```python
from build123d import *

# Parameters (mm, degrees)
F0_W           = 64
F0_H           = 25
F1_DEPTH       = 3
F3_D           = 3.3
F3_CSINK_D     = 6.72
F3_CSINK_ANGLE = 90
F4_R           = 5


with BuildPart() as f1:
    # F0 (on Front) → F1 (new body)
    with BuildSketch(Plane.XZ):
        with Locations((32, 12.5)):
            Rectangle(F0_W, F0_H)
    extrude(amount=F1_DEPTH)

    # F3 (through all)
    with Locations(Plane.XZ.offset(3)):
        with Locations((3, 21.5), (28, 21.5), (28, 3.5), (3, 3.5)):
            CounterSinkHole(F3_D / 2, F3_CSINK_D / 2, counter_sink_angle=F3_CSINK_ANGLE)

    # F4
    f4_edges = [f1.edges().sort_by_distance(p)[0] for p in [
        (64, -1.5, 0),
        (64, -1.5, 25),
    ]]
    fillet(f4_edges, radius=F4_R)


solid = f1.part
```
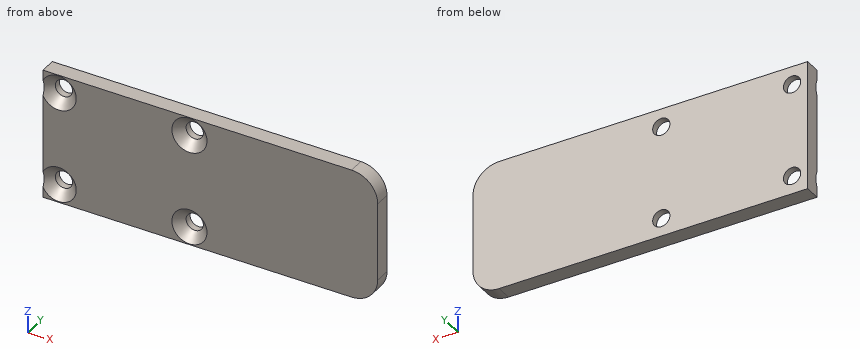
Could you check a few things on this model? Use its own coordinates, in mm. Coordinates: 2 decimals unless noted, no trailing zeros. Order: outer loops, then holes, each group sorted by start corner. A loop starts at its lowest first (then second) coordinate and runs counter-clockwise, first axis right, second up. Notation, with made-up numbers: M 50,34.25 L 82,34.25 A34 cw 82,71.25 Z; hole C 12,72.5 d1. An arc over 180 degrees is marked long. Use one line per item in the form item = value. Start each with the question number.
1. Suppose I cut it at B-B on z = 21.5. Write out the boundary of the cut face in (x, y).
2. Suppose I cut it at A-A on x = 3. Write out the boundary of the cut face in (y, z), then the cut area to 3 significant figures.
3. Please list where these lines run through material, in increasing order: line 1 (Z direction, x = 3, y = -0.95); line 2 (X direction, y = -2.2, z = 22.75); line 3 (X direction, y = -0.75, z = 3.5).
4. For pin 1 (3 mm diameter, centred on x = 28, z = 21.5, fed in from +Y); pin 2 (4 mm diameter, centred on x = 3, z = 3.5, fed in from -Y); pin 3 (5.5 mm diameter, centred on x = 3, z = 21.5, fed in from -Y), each with a flat end and sliding along its axis, tell me the tip position at first contact or that it passes through.
Geometry says:
q1.outline = M 0,-2.64 L 1.35,-1.29 L 1.35,0 L 0,0 Z; M 4.65,-1.29 L 6.36,-3 L 24.64,-3 L 26.35,-1.29 L 26.35,0 L 4.65,0 Z; M 29.65,-1.29 L 31.36,-3 L 63.77,-3 L 63.77,0 L 29.65,0 Z
q2.outline = M -3,0 L 0,0 L 0,1.85 L -1.29,1.85 L -3,0.14 Z; M -3,6.86 L -1.29,5.15 L 0,5.15 L 0,19.85 L -1.29,19.85 L -3,18.14 Z; M -3,24.86 L -1.29,23.15 L 0,23.15 L 0,25 L -3,25 Z
q2.area = 49.4 mm^2
q3.line_1 = 0 to 1.85, 5.15 to 19.85, 23.15 to 25
q3.line_2 = 0 to 0.77, 5.23 to 25.77, 30.23 to 63.18
q3.line_3 = 0 to 1.35, 4.65 to 26.35, 29.65 to 63.77
q4.pin_1 = through
q4.pin_2 = -1.64
q4.pin_3 = -2.39
